from build123d import *

# Parameters (mm, degrees)
BOSS_EXTRUDE2_DEPTH      = 19
BOSS_EXTRUDE2_DEPTH_BACK = 19
CUT_EXTRUDE2_START       = -14
CUT_EXTRUDE2_DEPTH       = 14


with BuildPart() as part:
    # Sketch3 → Boss-Extrude2 (new, two sides: drawn at the far end of the back side and taken through both)
    with BuildSketch(Plane.XY.offset(-BOSS_EXTRUDE2_DEPTH_BACK)):
        with BuildLine():
            Line((0, -38.1), (-66.04, -38.1))
            ThreePointArc((-66.04, -38.1), (-82.204461018, -31.404461018), (-88.9, -15.24))
            Line((-88.9, -15.24), (-88.9, 228.6))
            Line((-88.9, 228.6), (-79.97655577, 228.6))
            ThreePointArc((-79.97655577, 228.6), (-66.610078663, 224.284996353), (-58.289655577, 212.968966731))
            Line((-58.289655577, 212.968966731), (0, 38.1))
            ThreePointArc((0, 38.1), (38.1, 0), (0, -38.1))
        make_face()
    extrude(amount=BOSS_EXTRUDE2_DEPTH + BOSS_EXTRUDE2_DEPTH_BACK)

    # Sketch5 → Cut-Extrude2 (cut)
    with BuildSketch(Plane.XY.offset(19).offset(CUT_EXTRUDE2_START)):
        with BuildLine():
            Line((-38.1, 0), (-38.1, -38.1))
            Line((-38.1, -38.1), (0, -38.1))
            ThreePointArc((0, -38.1), (26.940768363, 26.940768363), (-38.1, 0))
        make_face()
    cut_extrude2 = extrude(amount=CUT_EXTRUDE2_DEPTH, mode=Mode.SUBTRACT)

    # Mirror2: Cut-Extrude2 across plane
    add(cut_extrude2.mirror(Plane.XY), mode=Mode.SUBTRACT)


solid = part.part
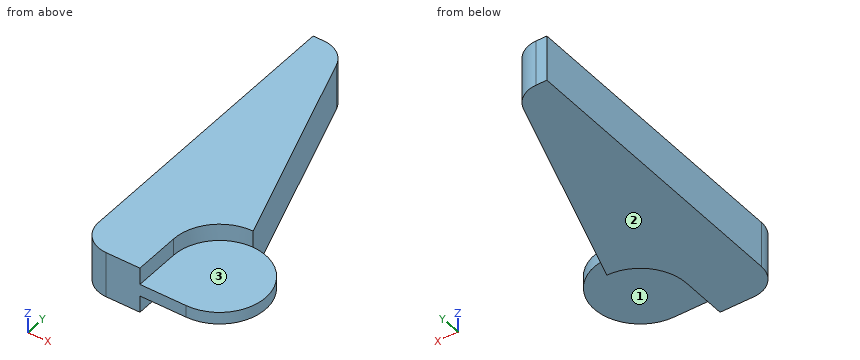
Input: part model. Units: mm. Frame: model coordinates. Face numbers are marked on the shaded views. A direction names the side the tool comes from. Coordinates: 2 decimals unless noted, no trailing zeros. Loops run counter-clockwise (first coordinate to the right, second up) from the corner with the lowest first, then second, coordinate; pieces in that order, holes last. Notation, with made-up numbers: (42.25, -33.5) -> (70.25, -33.5) arc R19 ccw to (70.25, -26.5) -> close; hole circle Ø6 at (89, 19.25). An arc over 180 degrees is marked (long way). Write item = value, one per line. Start each with the question number.
Item 1: Cut plane A-A, the plane z = -14. Return loops of the section in (x, y), plus the area to 3 significant figures.
Item 2: First-contact query: P1, Ø1, axis at x = 15.5, z = -4.5, coming from the +Y side; P2, Ø11, axis at y = -19.5, z = 14, coming from the +X side; P3, Ø5, axis at y = 120, z = -5, coming from the +X side. Flat tips, straight axial feed; report the tip coordinate or a pass-through.
Item 3: Cut plane B-B, the plane x = -34. Return loops of the section in (y, z).
Item 4: Cut plane D-D, the plane x = 20.5. Return loops of the section in (y, z), plus the area to 3 significant figures.
Item 5: Reachability of the marked faces 1, 2 and 3 from +Z, -Z, +X, -X, +Y, -Y: full face, straight path, thin tool, end or side. Return the list, or none.
Item 6: Material intervals for line 1 (Z direction, x = -8, y = -4.5); line 2 (X direction, y = 134.5, z = -15.5); line 3 (X direction, y = 161, z = -11.5), sorted ascending.
Item 7: Cut plane C-C, the plane x = 6. Return loops of the section in (y, z).
Ans:
q1.outline = (-88.9, -15.24) arc R22.86 ccw to (-66.04, -38.1) -> (-38.1, -38.1) -> (-38.1, 0) arc R38.1 cw to (0, 38.1) -> (-58.29, 212.97) arc R22.86 ccw to (-79.98, 228.6) -> (-88.9, 228.6) -> close
q1.area = 14,900 mm²
q2.P1 = 35.02
q2.P2 = -38.1
q2.P3 = -26.47
q3.outline = (-38.1, -5) -> (17.19, -5) -> (17.19, -19) -> (140.1, -19) -> (140.1, 19) -> (17.19, 19) -> (17.19, 5) -> (-38.1, 5) -> close
q4.outline = (-32.11, -5) -> (32.11, -5) -> (32.11, 5) -> (-32.11, 5) -> close
q4.area = 642 mm²
q5.face_1 = -Z, +X, -Y
q5.face_2 = -Z, +X, -X, +Y, -Y
q5.face_3 = +Z, +X, -Y
q6.line_1 = -5 to 5
q6.line_2 = -88.9 to -32.13
q6.line_3 = -88.9 to -40.97
q7.outline = (-37.62, -5) -> (37.62, -5) -> (37.62, 5) -> (-37.62, 5) -> close
